Autodesk Inventor part; units mm, degrees
ref_plane "YZ Plane" through (0, 0, 0) normal (1, 0, 0) x (0, 1, 0)
ref_plane "XZ Plane" through (0, 0, 0) normal (0, 1, 0) x (-1, 0, 0)
ref_plane "XY Plane" through (0, 0, 0) normal (0, 0, 1) x (1, 0, 0)
sketch "Sketch1" plane through (0, 0, 0) normal (0, 0, 1) x (1, 0, 0)
  circle A0 centre (0, 0) radius 25
  dimension "d0" = 50
extrude "Extrusion1" add sketch "Sketch1" along normal blind 10
sketch "Sketch2" plane through (0, 0, 10) normal (0, 0, 1) x (1, 0, 0)
  circle A0 centre (0, 0) radius 6.5
  dimension "d3" = 13
extrude "Extrusion2" add sketch "Sketch2" along normal blind 100
fillet "Fillet1" radius 1 1 edges at (-6.5, 0, 10)
sketch "Sketch4" plane through (0, 0, 0) normal (0, 0, -1) x (-1, 0, 0)
  arc A0 (19.3649, 5) -> (5, 19.3649) centre (0, 0) ccw
  line L0 (2.5, 17.4284) -> (2.5, 9.4868)
  line L1 (9.4868, 2.5) -> (17.4284, 2.5)
  arc A1 (5, 19.3649) -> (2.5, 17.4284) centre (4.5, 17.4284) ccw
  arc A2 (17.4284, 2.5) -> (19.3649, 5) centre (17.4284, 4.5) ccw
  arc A3 (2.5, 8.3666) -> (2.5153, 8.1193) centre (4.5, 8.3666) ccw
  arc A4 (8.1193, 2.5153) -> (8.3666, 2.5) centre (8.3666, 4.5) ccw
  arc A5 (7.6798, 3.6429) -> (3.6429, 7.6798) centre (0, 0) ccw
  arc A6 (2.5, 9.4868) -> (3.6429, 7.6798) centre (4.5, 9.4868) ccw
  arc A7 (7.6798, 3.6429) -> (9.4868, 2.5) centre (9.4868, 4.5) ccw
  point P0 (2.5, 19.8431)
  point P1 (19.8431, 2.5)
  point P2 (2.5, 7.0711)
  point P3 (7.0711, 2.5)
extrude "Extrusion3" cut sketch "Sketch4" against normal blind 10
pattern_circular "Circular Pattern1" count 4 over 360 about axis through (0, 0, 11) along (0, 0, -1) of "Extrusion3"
sketch "Sketch7" plane through (0, 0, 110) normal (0, 0, 1) x (1, 0, 0)
  circle A0 centre (0, 0) radius 7.5
  dimension "d38" = 15
extrude "Extrusion5" add sketch "Sketch7" along normal blind 384
sketch "Sketch8" plane through (0, 0, 494) normal (0, 0, 1) x (1, 0, 0)
  circle A0 centre (0, 0) radius 6.5
  dimension "d41" = 13
extrude "Extrusion6" add sketch "Sketch8" along normal blind 10
sketch "Sketch9" plane through (0, 0, 504) normal (0, 0, 1) x (1, 0, 0)
  circle A0 centre (0, 0) radius 10
  dimension "d44" = 20
extrude "Extrusion7" add sketch "Sketch9" along normal blind 2.5
thread "Thread1"
sketch "Sketch10" plane through (0, 0, 506.5) normal (0, 0, 1) x (1, 0, 0)
  circle A0 centre (0, 0) radius 10
extrude "Extrusion8" cut sketch "Sketch10" against normal blind 12.5
sketch "Sketch11" plane through (0, 0, 0) normal (0, 0, -1) x (-1, 0, 0)
  circle A0 centre (0, 0) radius 25
  circle A1 centre (0, 0) radius 25
extrude "Extrusion9" cut sketch "Sketch11" against normal blind 110
sketch "Sketch12" plane through (0, 0, 110) normal (0, 0, -1) x (-1, 0, 0)
  circle A0 centre (0, 0) radius 5
  dimension "d53" = 10
extrude "Extrusion10" add sketch "Sketch12" along normal blind 115
properties part number "leadscrew_latest_Y" material "Steel, Alloy"
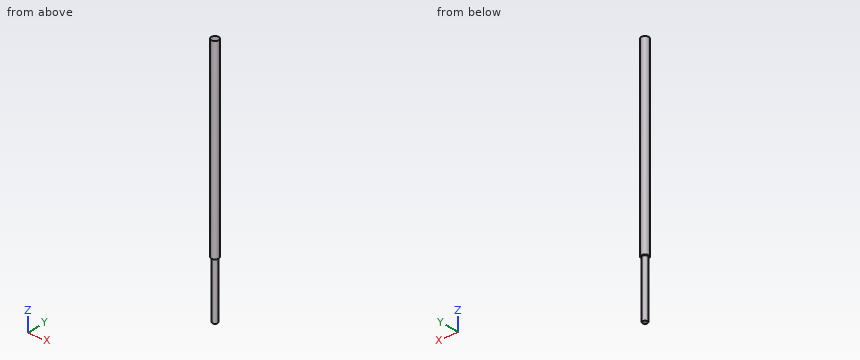
Design review of the part built by this model. Coordinates are the model's own, in mm. Coordinates: 2 decimals unless noted, no trailing zeros. Order: outer loops, then holes, each group sorted by start corner. A loop starts at its lowest first (then second) coordinate and runs counter-clockwise, first axis right, second up. Notation, with made-up numbers: (31, 32.5) - (64, 32.5) arc R30 ccw to (64, 68.5) - close; hole circle Ø11 at (38.25, 2). An arc over 180 degrees is marked (long way). Answer in a Markdown table with one row per item.
(1) Consider section A-A on x = 0. State the section outline as (y, z) points, plus the area to 3 significant figures.
Checked values:
| item | result |
|---|---|
| outline | (-7.5, 110) - (-5, 110) - (-5, -5) - (5, -5) - (5, 110) - (7.5, 110) - (7.5, 494) - (-7.5, 494) - close |
| area | 6,910 mm^2 |
(2) Consider section D-D on z = 256.5. State the section outline as (x, y) points, plus the area to 3 significant figures.
Checked values:
| item | result |
|---|---|
| outline | circle Ø15 at (0, 0) |
| area | 177 mm^2 |
(3) Clearance check with flat-ended pins moving along their axes: pin 1 (1 mm diameter, centred on y = -5.5, z = 434.5, fed in from +X); pin 2 (2 mm diameter, centred on y = 4, z = 211, fed in from -X); pin 3 (4 mm diameter, centred on y = 3, z = 372.5, fed in from +X). State where each tip first meets the part, or that it passes through.
Checked values:
| item | result |
|---|---|
| pin 1 | x = 5.59 |
| pin 2 | x = -6.87 |
| pin 3 | x = 7.43 |
(4) Consider section C-C on z = 56. State the section outline as (x, y) points, plus the area to 3 significant figures.
Checked values:
| item | result |
|---|---|
| outline | circle Ø10 at (0, 0) |
| area | 78.5 mm^2 |
(5) Wall thickness on line 1 along X through (y, z) = (0.25, 388.5); line 2 along Z through (x, y) = (-3.5, -5.75); line 3 along Y through (x, z) = (-0.5, 17): over which ranges is each line inside the solid? List them lowest first. Write a range as from..to.
Checked values:
| item | result |
|---|---|
| line 1 | -7.5..7.5 |
| line 2 | 110..494 |
| line 3 | -4.97..4.97 |
